Build history of the part. All positions in model axes, mm. Face numbers are marked on the shaded views. A direction names the side the tool comes from. Round coordinates to 2 decimals unless told otherwise and drop trailing zeros. Write each loop counter-clockwise with the first axis right and the second up, starting at its lowest first coordinate (ties: lowest second). Pieces come first, ordered by that corner, then holes. Notation, with made-up numbers: (-10.75, 74.5) -> (9.25, 74.5) arc R6 cw to (9.25, 85.5) -> close; hole circle Ø2 at (63, 10). An arc over 180 degrees is marked (long way). Return JSON: item names as keys, results as strings.
from build123d import *

# Parameters (mm, degrees)
BOSS_EXTRUDE1_DEPTH  = 114.3
SKETCH3_W            = 107.95
SKETCH3_H            = 109.22
CUT_EXTRUDE1_DEPTH   = 27.94
BOSS_EXTRUDE14_REACH = 32.48
SKETCH4_R            = 2.032
SKETCH5_R            = 2.032
SKETCH5_R_2          = 11.176
SKETCH5_R_3          = 1.27
CUT_EXTRUDE2_DEPTH   = 2.54
SKETCH7_R            = 12.319
BOSS_EXTRUDE15_DEPTH = 24.5
CUT_EXTRUDE3_REACH   = 143.34
SKETCH8_R            = 10.287
BOSS_EXTRUDE17_DEPTH = 5.08
SKETCH16_R           = 14.6685
SKETCH16_R_2         = 13.1445
BOSS_EXTRUDE18_DEPTH = 8.128


with BuildPart() as part:
    # Sketch1 → Boss-Extrude1 (new body)
    with BuildSketch(Plane.XY):
        Polygon((0, 0), (0, 88.9), (-6.35, 88.9), (-6.35, -30.48), (110.49, -30.48), (110.49, 0), align=None)
    extrude(amount=BOSS_EXTRUDE1_DEPTH)

    # Sketch3 → Cut-Extrude1 (cut)
    with BuildSketch(Plane(origin=(0, 0, 0), x_dir=(1, 0, 0), z_dir=(0, 1, 0))):
        with Locations((53.975, -57.15)):
            Rectangle(SKETCH3_W, SKETCH3_H)
    extrude(amount=-CUT_EXTRUDE1_DEPTH, mode=Mode.SUBTRACT)

    # Sketch4 → Boss-Extrude14 (add, up to next)
    with BuildSketch(Plane(origin=(0, 0, 0), x_dir=(1, 0, 0), z_dir=(0, 1, 0)), mode=Mode.PRIVATE) as boss_extrude14_sk1:
        with BuildLine():
            Line((0, -2.54), (6.35, -2.54))
            Line((6.35, -2.54), (6.35, -6.35))
            ThreePointArc((6.35, -6.35), (5.606051224, -8.146051224), (3.81, -8.89))
            Line((3.81, -8.89), (0, -8.89))
            Line((0, -8.89), (0, -2.54))
        make_face()
        with Locations((2.54, -4.826)):
            Circle(SKETCH4_R, mode=Mode.SUBTRACT)
    boss_extrude14_tool1 = extrude(boss_extrude14_sk1.sketch, amount=-BOSS_EXTRUDE14_REACH, mode=Mode.PRIVATE) - part.part
    add(boss_extrude14_tool1.solids().sort_by_distance((3.175, 0, 2.629803))[0])
    # Sketch4 → Boss-Extrude14 (add, up to next)
    with BuildSketch(Plane(origin=(0, 0, 0), x_dir=(1, 0, 0), z_dir=(0, 1, 0)), mode=Mode.PRIVATE) as boss_extrude14_sk2:
        with BuildLine():
            Line((101.6, -2.54), (101.6, -6.35))
            ThreePointArc((101.6, -6.35), (102.343948776, -8.146051224), (104.14, -8.89))
            Line((104.14, -8.89), (107.95, -8.89))
            Line((107.95, -8.89), (107.95, -2.54))
            Line((107.95, -2.54), (101.6, -2.54))
        make_face()
        with Locations((105.41, -4.826)):
            Circle(SKETCH4_R, mode=Mode.SUBTRACT)
    boss_extrude14_tool2 = extrude(boss_extrude14_sk2.sketch, amount=-BOSS_EXTRUDE14_REACH, mode=Mode.PRIVATE) - part.part
    add(boss_extrude14_tool2.solids().sort_by_distance((101.689803, 0, 4.445))[0])
    # Sketch4 → Boss-Extrude14 (add, up to next)
    with BuildSketch(Plane(origin=(0, 0, 0), x_dir=(1, 0, 0), z_dir=(0, 1, 0)), mode=Mode.PRIVATE) as boss_extrude14_sk3:
        with BuildLine():
            Line((107.95, -111.76), (101.6, -111.76))
            Line((101.6, -111.76), (101.6, -107.95))
            ThreePointArc((101.6, -107.95), (102.343948776, -106.153948776), (104.14, -105.41))
            Line((104.14, -105.41), (107.95, -105.41))
            Line((107.95, -105.41), (107.95, -111.76))
        make_face()
        with Locations((105.41, -109.474)):
            Circle(SKETCH4_R, mode=Mode.SUBTRACT)
    boss_extrude14_tool3 = extrude(boss_extrude14_sk3.sketch, amount=-BOSS_EXTRUDE14_REACH, mode=Mode.PRIVATE) - part.part
    add(boss_extrude14_tool3.solids().sort_by_distance((104.775, 0, 111.670197))[0])
    # Sketch4 → Boss-Extrude14 (add, up to next)
    with BuildSketch(Plane(origin=(0, 0, 0), x_dir=(1, 0, 0), z_dir=(0, 1, 0)), mode=Mode.PRIVATE) as boss_extrude14_sk4:
        with BuildLine():
            Line((6.35, -111.76), (6.35, -107.95))
            ThreePointArc((6.35, -107.95), (5.606051224, -106.153948776), (3.81, -105.41))
            Line((3.81, -105.41), (0, -105.41))
            Line((0, -105.41), (0, -111.76))
            Line((0, -111.76), (6.35, -111.76))
        make_face()
        with Locations((2.54, -109.474)):
            Circle(SKETCH4_R, mode=Mode.SUBTRACT)
    boss_extrude14_tool4 = extrude(boss_extrude14_sk4.sketch, amount=-BOSS_EXTRUDE14_REACH, mode=Mode.PRIVATE) - part.part
    add(boss_extrude14_tool4.solids().sort_by_distance((6.260197, 0, 109.855))[0])

    # Sketch5 → Cut-Extrude2 (cut)
    with BuildSketch(Plane.XZ.offset(30.48)):
        with Locations((7.62, 73.787)):
            Circle(SKETCH5_R)
        with Locations((40.894, 73.787)):
            Circle(SKETCH5_R)
        with Locations((40.894, 40.513)):
            Circle(SKETCH5_R)
        with Locations((7.62, 40.513)):
            Circle(SKETCH5_R)
        with Locations((24.13, 57.15)):
            Circle(SKETCH5_R_2)
        with Locations((51.308, 57.15)):
            Circle(SKETCH5_R_3)
    extrude(amount=-CUT_EXTRUDE2_DEPTH, mode=Mode.SUBTRACT)

    # Sketch7 → Boss-Extrude15 (add)
    with BuildSketch(Plane.ZY.offset(6.35)):
        with Locations((57.15, 38.1)):
            Circle(SKETCH7_R)
    extrude(amount=BOSS_EXTRUDE15_DEPTH)

    # Sketch8 → Cut-Extrude3 (cut, up to next)
    with BuildSketch(Plane.ZY.offset(30.85), mode=Mode.PRIVATE) as cut_extrude3_sk1:
        with Locations((57.15, 38.1)):
            Circle(SKETCH8_R)
    cut_extrude3_tool1 = extrude(cut_extrude3_sk1.sketch, amount=-CUT_EXTRUDE3_REACH, mode=Mode.PRIVATE) & part.part
    add(cut_extrude3_tool1.solids().sort_by_distance((-30.85, 38.1, 57.15))[0], mode=Mode.SUBTRACT)

    # Sketch11 → Boss-Extrude17 (add)
    with BuildSketch(Plane.ZY.offset(6.35)):
        with BuildLine():
            Line((54.737, 50.180363902), (54.737, 53.307305955))
            Line((54.737, 53.307305955), (59.563, 53.307305955))
            Line((59.563, 53.307305955), (59.563, 50.180363902))
            ThreePointArc((59.563, 50.180363902), (57.15, 50.419), (54.737, 50.180363902))
        make_face()
    extrude(amount=BOSS_EXTRUDE17_DEPTH)

    # Sketch16 → Boss-Extrude18 (add)
    with BuildSketch(Plane(origin=(0, -27.94, 0), x_dir=(1, 0, 0), z_dir=(0, 1, 0))):
        with Locations((51.308, -57.15)):
            Circle(SKETCH16_R)
        with Locations((51.308, -57.15)):
            Circle(SKETCH16_R_2, mode=Mode.SUBTRACT)
    extrude(amount=BOSS_EXTRUDE18_DEPTH)


solid = part.part
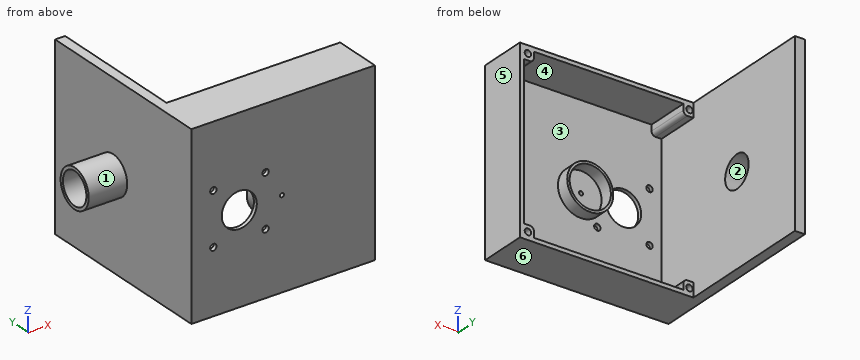
Q1. Wall check: L1, parallel to Z at x = 2.54, y = -18.25; L2, parallel to X at y = -10.5, z = 99; L3, parallel to X at y = -29, z = 57 (3 decimals). Give the ranges that are in metal, low to high.
Verdict:
{"L1": "z = 0 to 2.79, 6.86 to 8.89, 105.41 to 107.44, 111.51 to 114.3", "L2": "x = -6.35 to 0, 107.95 to 110.49", "L3": "x = -6.35 to 12.955, 35.305 to 50.047, 52.569 to 110.49"}
Q2. Saw through at C-C on z = 89.5. List the corners of the cut face in (x, y).
Verdict:
{"outline": "(-6.35, -30.48) -> (110.49, -30.48) -> (110.49, 0) -> (107.95, 0) -> (107.95, -27.94) -> (0, -27.94) -> (0, 88.9) -> (-6.35, 88.9) -> close"}
Q3. Two-plate mould, pull along X, no slides. Class the marked faces 4, 5 and 6: +X half, -X half, draft (parallel to the pull), parting line (faces both ways), or undercut.
Verdict:
{"face 4": "undercut", "face 5": "+X half", "face 6": "draft"}
Q4. 3-axis set-ups, long thin cutter, end or side, ignore diameter. For the marked faces 1, 2 and 3: which of +Z, -Z, +X, -X, +Y, -Y reach the whole face in a straight line?
Verdict:
{"face 1": "-X", "face 2": "+X, -X", "face 3": "+Y"}
Q5. Pin check, flat tips, straight feed: pin 1 Ø1.5 at (y, z) = (38.5, 66) entering from +X; pin 2 Ø1.9 at (y, z) = (-11, 5.5) entering from -X; pin 3 Ø3 at (y, z) = (41, 13.5) entering from +X; pin 4 Ø6.5 at (x, z) = (7.62, 73.787) entering from +Y. Stop position of each tip, or through.
Verdict:
{"pin 1": "passes through", "pin 2": "stops at x = -6.35", "pin 3": "stops at x = 0", "pin 4": "stops at y = -27.94"}
Q6. Saw through at A-A on x = 24.13. List the corners of the cut face in (y, z).
Verdict:
{"outline": "(-30.48, 0) -> (0, 0) -> (0, 2.54) -> (-27.94, 2.54) -> (-27.94, 45.97) -> (-30.48, 45.97) -> close; (-30.48, 68.33) -> (-27.94, 68.33) -> (-27.94, 111.76) -> (0, 111.76) -> (0, 114.3) -> (-30.48, 114.3) -> close"}
Q7. Saw through at D-D on x = 86. List the corners of the cut face in (y, z).
Verdict:
{"outline": "(-30.48, 0) -> (0, 0) -> (0, 2.54) -> (-27.94, 2.54) -> (-27.94, 111.76) -> (0, 111.76) -> (0, 114.3) -> (-30.48, 114.3) -> close"}
Q8. Saw through at B-B on y = 38.1. List the corners of the cut face in (x, z), then the cut area to 3 significant figures.
Verdict:
{"outline": "(-30.85, 44.83) -> (-6.35, 44.83) -> (-6.35, 0) -> (0, 0) -> (0, 46.86) -> (-30.85, 46.86) -> close; (-30.85, 67.44) -> (0, 67.44) -> (0, 114.3) -> (-6.35, 114.3) -> (-6.35, 69.47) -> (-30.85, 69.47) -> close", "area": "695 mm²"}
